```python
from build123d import *

# Parameters (mm, degrees)
SKETCH1_R           = 27.051
SKETCH1_R_2         = 24.511
BOSS_EXTRUDE1_DEPTH = 1111.25
SKETCH2_W           = 2.54
SKETCH2_H           = 1.397
SKETCH11_W          = 1.796741038
SKETCH11_H          = 1.524


with BuildPart() as part:
    # Sketch1 → Boss-Extrude1 (new body)
    with BuildSketch(Plane(origin=(0, 0, 0), x_dir=(1, 0, 0), z_dir=(0, 1, 0))):
        Circle(SKETCH1_R)
        Circle(SKETCH1_R_2, mode=Mode.SUBTRACT)
    extrude(amount=BOSS_EXTRUDE1_DEPTH)

    # Sketch2 → Cut-Revolve1 (revolve, cut)
    with BuildSketch(Plane.XY):
        with Locations((24.003, 6.9215)):
            Rectangle(SKETCH2_W, SKETCH2_H)
    cut_revolve1 = revolve(axis=Axis((0, 1111.25, 0), (0, -1, 0)), mode=Mode.SUBTRACT)

    # Mirror1: Cut-Revolve1 across plane
    add(cut_revolve1.mirror(Plane(origin=(0, 555.625, 0), x_dir=(0, 0, 1), z_dir=(0, -1, 0))), mode=Mode.SUBTRACT)

    # Sketch11 → Cut-Revolve3 (revolve, cut)
    with BuildSketch(Plane.XY):
        with Locations((26.806370519, 11.684)):
            Rectangle(SKETCH11_W, SKETCH11_H)
    revolve(axis=Axis((0, 1111.25, 0), (0, -1, 0)), mode=Mode.SUBTRACT)


solid = part.part
```
CAD build for the part. Positions are in the model's coordinates, mm. A direction names the side the tool comes from. Round coordinates to 2 decimals unless told otherwise and drop trailing zeros. Write each loop counter-clockwise with the first axis right and the second up, starting at its lowest first coordinate (ties: lowest second). Pieces come first, ordered by that corner, then holes. Notation, with made-up numbers: (71, 18.5) - (89, 18.5) arc R6 cw to (89, 23.5) - close; hole circle Ø9 at (-22, -20.75). An arc over 180 degrees is marked (long way). Write item = value, one per line. Start each with the question number.
Q1. Probe L1, parallel to Z at x = 0, y = 3.5; L2, parallel to Y at x = -19, z = -18; L3, parallel to X at y = 767.5, z = 1. List the from-to ranges inside material, lowest first. Write a range as from..to.
Q2. Mould opens along Z. For faces 3 (the flat face through (-14, 10.922, -22)), 4 (the flat face through (21, 1105.027, 13)), 5 (the cylindrical face through (25.8, 554.16, -8.13)) say: pulls with the +Z half, pulls with the -Z half, needs draft (parallel to the pull), parting line crosses it, or undercut.
Q3. Drop flat-ended pins along their axis: pin 1 (2 mm diameter, centred on x = 10.5, y = 197, fed in from +Z); pin 2 (2 mm diameter, centred on y = 978.5, z = 6, fed in from -X); pin 3 (12 mm diameter, centred on y = 378, z = -8.5, fed in from +X). Give the stop position or say it passes through.
Q4. Which spindle directions (+Z, -Z, +X, -X, +Y, -Y) get a long thin tool onto all of the face, cutting with end or side? Do faces 1 (the cylindrical face through (-19.451, 547.953, 14.915)), 2 (the flat face through (21, 7.62, 13)). Say none if no direction does.
Q5. Band-saw the part on C-C (y = 520.5). Give the cut face in (x, z).
Answers below:
q1.L1 = -27.05..-24.51, 24.51..27.05
q1.L2 = 0..10.92, 12.45..1111.25
q1.L3 = -27.03..-24.49, 24.49..27.03
q2.face_3 = needs draft
q2.face_4 = undercut
q2.face_5 = parting line crosses it
q3.pin_1 = 25.33
q3.pin_2 = -26.58
q3.pin_3 = 26.94
q4.face_1 = +Y, -Y
q4.face_2 = none
q5.outline = circle Ø54.1 at (0, 0); hole circle Ø49.02 at (0, 0)
